from build123d import *

# Parameters (mm, degrees)
EXTRUDE_THIN1_DEPTH      = 675
EXTRUDE_THIN1_DEPTH_BACK = 675
SKETCH4_R                = 8.2
CUT_EXTRUDE3_DEPTH       = 110
SKETCH5_R                = 8.2
CUT_EXTRUDE4_DEPTH       = 110


with BuildPart() as part:
    # Sketch1 → Extrude-Thin1 (new, two sides: drawn at the far end of the back side and taken through both)
    with BuildSketch(Plane(origin=(0, 0, 0), x_dir=(0, 0, -1), z_dir=(1, 0, 0)).offset(-EXTRUDE_THIN1_DEPTH_BACK)):
        with BuildLine():
            Line((-30, 52), (-30, -52))
            ThreePointArc((-30, -52), (-27.656854249, -57.656854249), (-22, -60))
            Line((-22, -60), (22, -60))
            ThreePointArc((22, -60), (27.656854249, -57.656854249), (30, -52))
            Line((30, -52), (30, 52))
            ThreePointArc((30, 52), (27.656854249, 57.656854249), (22, 60))
            Line((22, 60), (-22, 60))
            ThreePointArc((-22, 60), (-27.656854249, 57.656854249), (-30, 52))
        make_face()
        with BuildLine():
            Line((-27, 52), (-27, -52))
            ThreePointArc((-27, -52), (-25.535533906, -55.535533906), (-22, -57))
            Line((-22, -57), (22, -57))
            ThreePointArc((22, -57), (25.535533906, -55.535533906), (27, -52))
            Line((27, -52), (27, 52))
            ThreePointArc((27, 52), (25.535533906, 55.535533906), (22, 57))
            Line((22, 57), (-22, 57))
            ThreePointArc((-22, 57), (-25.535533906, 55.535533906), (-27, 52))
        make_face(mode=Mode.SUBTRACT)
    extrude(amount=EXTRUDE_THIN1_DEPTH + EXTRUDE_THIN1_DEPTH_BACK)

    # Sketch4 → Cut-Extrude3 (cut)
    with BuildSketch(Plane.XY.offset(30)):
        with Locations(Location((0, 0, 0), (0, 0, 180))):
            Circle(SKETCH4_R)
    extrude(amount=-CUT_EXTRUDE3_DEPTH, mode=Mode.SUBTRACT)

    # Sketch5 → Cut-Extrude4 (cut)
    with BuildSketch(Plane(origin=(0, -1598, -30), x_dir=(1, 0, 0), z_dir=(0, 0, 1))):
        with Locations(Location((350, 1598, 0), (0, 0, 180))):
            Circle(SKETCH5_R)
        with Locations(Location((530, 1598, 0), (0, 0, 180))):
            Circle(SKETCH5_R)
        with Locations(Location((-350, 1598, 0), (0, 0, 180))):
            Circle(SKETCH5_R)
        with Locations(Location((-530, 1598, 0), (0, 0, 180))):
            Circle(SKETCH5_R)
    extrude(amount=CUT_EXTRUDE4_DEPTH, mode=Mode.SUBTRACT)


solid = part.part
Here's how the part is built. I have some questions about the finished solid (model axes, mm). A direction names the side the tool comes from. Give positions to 0.01 mm unless a question says otherwise; leave off trailing zeros. Order: outer loops, then holes, each group sorted by start corner. A loop starts at its lowest first (then second) coordinate and runs counter-clockwise, first axis right, second up. Notation, with made-up numbers: (-38.5, 2.5) -> (-14.5, 2.5) arc R29 ccw to (-14.5, 40.5) -> close; hole circle Ø2 at (46, -34.75). An arc over 180 degrees is marked (long way). Use a Markdown table: item, result. Add a question column.
Item 1: Imagine slicing it at B-B on z = 9.5. Please give me the cut outline in (x, y).
Item 2: For faces 4 (the face through (-9, 57, 0)), 5 (the face through (-9, 60, 0)), which set-ups out of +Z, -Z, +X, -X, +Y, -Y let a thin tool reach every point of the face, with its end or its side?
Item 3: I need wall thicknesses on line 1 (Y direction, x = 121, z = -15.5); line 2 (Z direction, x = 315, y = 10.5); line 3 (Y direction, x = 530, z = -28.4). Which ranges of each line are inside material? Lowest first, please.
Item 4: Imagine slicing it at A-A on y = 37. Please give me the cut outline in (x, z).
Item 5: If we mould it in two halves opening along Z, with no side actions, what happens to faces 1 (the face through (-9, -57, 0)), 2 (the face through (-9, -1, -30)), 3 (the face through (-675, 0, 29))? For each: pulls with the +Z half, pulls with the -Z half, needs draft (parallel to the pull), parting line crosses it, or undercut.
Item 6: Imagine slicing it at C-C on x = 58.5. Please give me the cut outline in (y, z).
Item 7: Will these pins go through, and if not, where does the flat tip stop? pin 1 (19 mm diameter, centred on x = 350, y = 0, fed in from -Z); pin 2 (15 mm diameter, centred on x = -350, y = 0, fed in from -Z).
Data:
| question | item | result |
|---|---|---|
| 1 | outline | (-675, -60) -> (675, -60) -> (675, -57) -> (-675, -57) -> close; (-675, 57) -> (675, 57) -> (675, 60) -> (-675, 60) -> close |
| 2 | face 4 | +X, -X |
| 2 | face 5 | +Z, -Z, +X, -X, +Y |
| 3 | line 1 | y = -60 to -57, 57 to 60 |
| 3 | line 2 | z = -30 to -27, 27 to 30 |
| 3 | line 3 | y = -56.8 to -8.2, 8.2 to 56.8 |
| 4 | outline | (-675, -30) -> (675, -30) -> (675, -27) -> (-675, -27) -> close; (-675, 27) -> (675, 27) -> (675, 30) -> (-675, 30) -> close |
| 5 | face 1 | undercut |
| 5 | face 2 | pulls with the -Z half |
| 5 | face 3 | needs draft |
| 6 | outline | (-60, -22) arc R8 ccw to (-52, -30) -> (52, -30) arc R8 ccw to (60, -22) -> (60, 22) arc R8 ccw to (52, 30) -> (-52, 30) arc R8 ccw to (-60, 22) -> close; hole (-57, -22) arc R5 ccw to (-52, -27) -> (52, -27) arc R5 ccw to (57, -22) -> (57, 22) arc R5 ccw to (52, 27) -> (-52, 27) arc R5 ccw to (-57, 22) -> close |
| 7 | pin 1 | stops at z = -30 |
| 7 | pin 2 | passes through |
